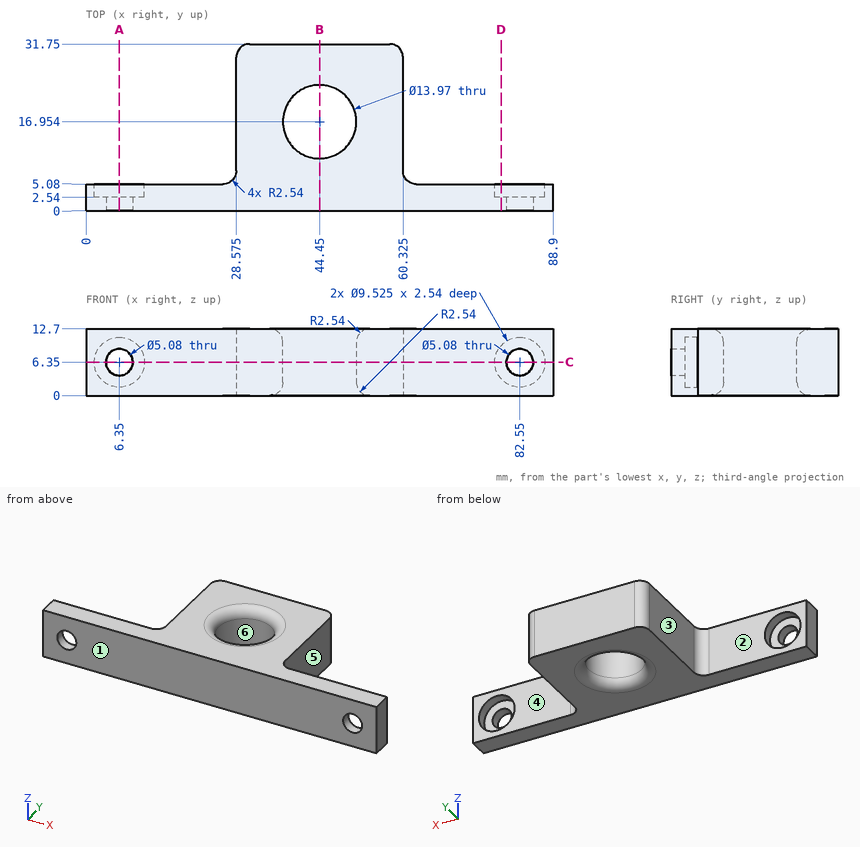
Design review of the part shown in the three views and the two pictorial views. Dimensions are in mm from the part's minimum x, y and z. A direction names the side the tool comes from. Round coordinates to 2 decimals unless told otherwise and drop trailing zeros. Loops run counter-clockwise (first coordinate to the right, second up) from the corner with the lowest first, then second, coordinate; pieces in that order, holes last. Notation, with made-up numbers: (28.5, 72) -> (65.5, 72) arc R32 ccw to (65.5, 99) -> close; hole circle Ø3 at (84.25, 64). An arc over 180 degrees is marked (long way). Answer as CSV lines item,"result".
1) Tool access review of the marked faces 1 and 2: name each direction out of +Z, -Z, +X, -X, +Y, -Y from which nothing blocks a thin tool from reaching the whole face with its end or side.
Geometry results:
face 1,"+Z, -Z, +X, -X, -Y"
face 2,"+Z, -Z, -X, +Y"
2) To check wall thickness, follow line 1 along X through (y, z) = (0.8, 6.35); line 2 along X through (y, z) = (3.9, 6.35); line 3 along Z through (x, y) = (6, 4). State the ranges of each line that lie inside material, in increasing order. Write a range as from..to.
Geometry results:
line 1,"x = 0..3.81, 8.89..80.01, 85.09..88.9"
line 2,"x = 0..1.59, 11.11..77.79, 87.31..88.9"
line 3,"z = 0..1.6, 11.1..12.7"
3) For P1, Ø6.5, axis at y = 19, z = 6, coming from the -X side (1 decimal); P2, Ø3, axis at x = 4.5, z = 6, coming from the +Y side; P3, Ø4, axis at x = 22, z = 2, coming from the +Y side, all flat-tipped, find the tip position at first contact; note any pin that passes through.
Geometry results:
P1,"stops at x = 28.6"
P2,"stops at y = 2.54"
P3,"stops at y = 5.08"
4) Add section C-C on z = 6.35. State how many separate pieces and enclosed holes the cut face has, plus the area to 3 significant figures.
Geometry results:
separate pieces,"3"
enclosed holes,"1"
area,"1,070 mm²"
5) Add section A-A on x = 6.35. Write out the cut boundary in (y, z).
Geometry results:
outline,"(0, 0) -> (5.08, 0) -> (5.08, 1.59) -> (2.54, 1.59) -> (2.54, 3.81) -> (0, 3.81) -> close; (0, 8.89) -> (2.54, 8.89) -> (2.54, 11.11) -> (5.08, 11.11) -> (5.08, 12.7) -> (0, 12.7) -> close"
6) Draft analysis for pull direction X (two halves, no side actions). For the marked faces 3, 4, 5 and 6, state which applies: pulls with the +X half, pulls with the -X half, needs draft (parallel to the pull), parting line crosses it, or undercut.
Geometry results:
face 3,"pulls with the -X half"
face 4,"needs draft"
face 5,"pulls with the +X half"
face 6,"undercut"
7) Add section B-B on x = 44.45. Write out the cut boundary in (y, z), plus the area to 3 significant figures.
Geometry results:
outline,"(0, 0) -> (7.43, 0) arc R2.54 ccw to (9.97, 2.54) -> (9.97, 10.16) arc R2.54 ccw to (7.43, 12.7) -> (0, 12.7) -> close; (23.94, 2.54) arc R2.54 ccw to (26.48, 0) -> (31.75, 0) -> (31.75, 12.7) -> (26.48, 12.7) arc R2.54 ccw to (23.94, 10.16) -> close"
area,"220 mm²"
8) Add section D-D on x = 79. Write out the cut boundary in (y, z) (1 decimal).
Geometry results:
outline,"(0, 0) -> (5.1, 0) -> (5.1, 3.2) -> (2.5, 3.2) -> (2.5, 9.5) -> (5.1, 9.5) -> (5.1, 12.7) -> (0, 12.7) -> close"
